Drawing for the job (mm, zero at the part's lowest x, y, z). A direction names the side the tool comes from. Coordinates: 2 decimals unless noted, no trailing zeros. Order: outer loops, then holes, each group sorted by start corner. A loop starts at its lowest first (then second) coordinate and runs counter-clockwise, first axis right, second up.
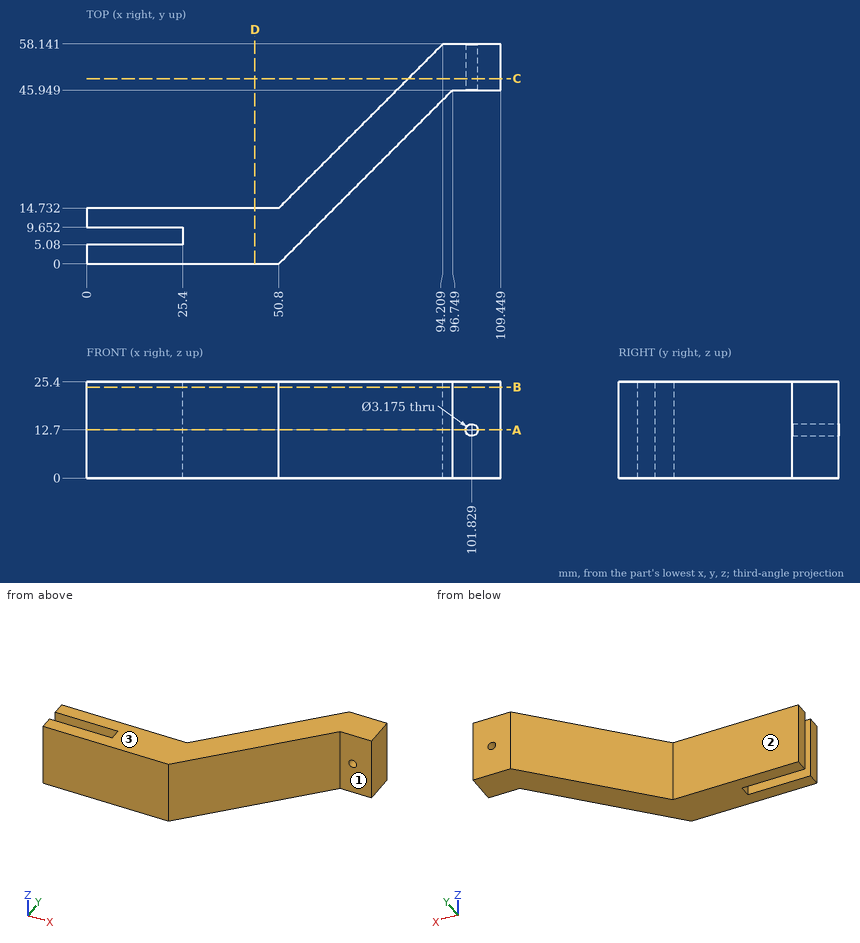
(1) Slice it at A-A, the plane z = 12.7. Give the cut face in (x, y), then the cut area to 3 significant figures.
(2) Slice it at B-B, the plane z = 24. Give the cut face in (x, y), then the cut area to 3 significant figures.
(3) Probe line 1 (Y direction, x = 22.5, z = 24); line 2 (Y direction, x = 66.5, z = 2.75); line 3 (Y direction, x = 32.5, z = 10.25). List the from-to ranges inside material, lowest first.
(4) Slice it at D-D, the plane x = 44.5. Give the cut face in (y, z).
(5) Slice it at C-C, the plane y = 49. Give the cut face in (x, z) (1 decimal), then the cut area to 3 significant figures.
(6) Tool access for the marked faces 1, 2 and 3: list every direction of +Z, -Z, +X, -X, +Y, -Y with a clear straight run to the whole face (end or side of a thin tool).
(7) Drop flat-ended pins along their axis: pin 1 (12.5 mm diameter, centred on x = 16.5, z = 14, fed in from +Y); pin 2 (4 mm diameter, centred on x = 96.5, z = 20, fed in from -Y); pin 3 (14 mm diameter, centred on x = 105.5, z = 12.5, fed in from -Y). Give the stop position or say it passes through.
Here are the results:
1. outline: (0, 0) - (50.8, 0) - (96.75, 45.95) - (100.24, 45.95) - (100.24, 58.14) - (94.21, 58.14) - (50.8, 14.73) - (0, 14.73) - (0, 9.65) - (25.4, 9.65) - (25.4, 5.08) - (0, 5.08) - close; (103.42, 45.95) - (109.45, 45.95) - (109.45, 58.14) - (103.42, 58.14) - close
1. area: 1,420 mm2
2. outline: (0, 0) - (50.8, 0) - (96.75, 45.95) - (109.45, 45.95) - (109.45, 58.14) - (94.21, 58.14) - (50.8, 14.73) - (0, 14.73) - (0, 9.65) - (25.4, 9.65) - (25.4, 5.08) - (0, 5.08) - close
2. area: 1,460 mm2
3. line 1: y = 0 to 5.08, 9.65 to 14.73
3. line 2: y = 15.7 to 30.43
3. line 3: y = 0 to 14.73
4. outline: (0, 0) - (14.73, 0) - (14.73, 25.4) - (0, 25.4) - close
5. outline: (85.1, 0) - (109.4, 0) - (109.4, 25.4) - (85.1, 25.4) - close; hole circle Ø3.2 at (101.8, 12.7)
5. area: 611 mm2
6. face 1: +Z, -Z, +X, -Y
6. face 2: +Z, -Z, -X, +Y
6. face 3: +Z, +X, -X, +Y, -Y
7. pin 1: stops at y = 14.73
7. pin 2: stops at y = 43.7
7. pin 3: stops at y = 45.95
